Check sheet for the modelled part. Datum: model origin and axes. Units: mm. Face numbers are marked on the shaded views. A direction names the side the tool comes from. Round coordinates to 2 decimals unless told otherwise and drop trailing zeros. One line per item, written item: value. Start each with the question number.
1. Go/stop test with flat-tipped pins: pin 1 (3 mm diameter, centred on x = 4, z = 2.5, fed in from +Y); pin 2 (0.6 mm diameter, centred on x = 2.5, y = -7, fed in from -Z); pin 3 (1.5 mm diameter, centred on y = 2, z = 1.5, fed in from -X). Record where each tip stops, or that it passes through.
2. Material ranges on L1, parallel to Z at x = -5.25, y = -8; L2, parallel to X at y = 0.75, z = 4; L3, parallel to Y at x = 0, z = -0.9, recorded low to high.
3. Set-up check for the marked faces 1, 2 and 3: record each of +Z, -Z, +X, -X, +Y, -Y from which the full face is reachable in a straight line by a thin tool's end or side.
4. Release check for a two-part mould opening along X. For the marked faces 4, 5 and 6 record: +X half, -X half, draft (parallel to the pull), parting line (faces both ways), or undercut.
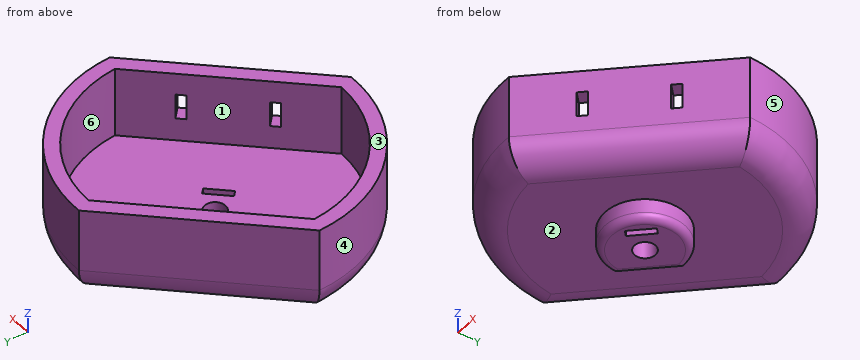
from build123d import *

# Parameters (mm, degrees)
BOSS_EXTRUDE1_DEPTH = 5
BOSS_EXTRUDE2_START = 1.5
BOSS_EXTRUDE2_DEPTH = 1.5
FILLET1_R           = 2
BOSS_EXTRUDE3_DEPTH = 1.5
SKETCH4_R           = 0.75
CUT_EXTRUDE1_DEPTH  = 17.248076932
SKETCH5_W           = 1.787924943
SKETCH5_H           = 0.660460042
CUT_EXTRUDE2_DEPTH  = 1
FILLET2_R           = 0.5


with BuildPart() as part:
    # Sketch1 → Boss-Extrude1 (new body)
    with BuildSketch(Plane.XY):
        with BuildLine():
            Line((0, 10), (-9.999822986, 0.0595))
            ThreePointArc((-9.999822986, 0.0595), (-7.09207304, -7.05), (0, -10))
            Line((0, -10), (10, 0))
            ThreePointArc((10, 0), (7.071067812, 7.071067812), (0, 10))
        make_face()
        with BuildLine():
            Line((0.403373919, 8.990955983), (-8.993196905, -0.349870591))
            ThreePointArc((-8.993196905, -0.349870591), (-6.383472043, -6.344390016), (-0.405092287, -8.990878725))
            Line((-0.405092287, -8.990878725), (8.990878725, 0.405092287))
            ThreePointArc((8.990878725, 0.405092287), (6.363352853, 6.36456915), (0.403373919, 8.990955983))
        make_face(mode=Mode.SUBTRACT)
    extrude(amount=BOSS_EXTRUDE1_DEPTH)

    # Sketch2 → Boss-Extrude2 (add)
    with BuildSketch(Plane(origin=(0, 0, 0), x_dir=(-1, 0, 0), z_dir=(0, 0, -1)).offset(BOSS_EXTRUDE2_START)):
        with BuildLine():
            Line((0, 10), (9.999822986, 0.0595))
            ThreePointArc((9.999822986, 0.0595), (7.09207304, -7.05), (0, -10))
            Line((0, -10), (-10, 0))
            ThreePointArc((-10, 0), (-7.071067812, 7.071067812), (0, 10))
        make_face()
    extrude(amount=-BOSS_EXTRUDE2_DEPTH)

    # Fillet1
    fillet1_edges = [part.edges().sort_by_distance(p)[0] for p in [
        (7.071067812, 7.071067812, -1.5),
        (5, -5, -1.5),
        (-7.09207304, -7.05, -1.5),
        (-4.999911493, 5.02975, -1.5),
    ]]
    fillet(fillet1_edges, radius=FILLET1_R)

    # Sketch3 → Boss-Extrude3 (add)
    with BuildSketch(Plane(origin=(0, 0, -1.5), x_dir=(-1, 0, 0), z_dir=(0, 0, -1))):
        with BuildLine():
            Line((0, 2.854684063), (2.854684063, 0))
            ThreePointArc((2.854684063, 0), (-2.018566459, -2.018566459), (0, 2.854684063))
        make_face()
    extrude(amount=BOSS_EXTRUDE3_DEPTH)

    # Sketch4 → Cut-Extrude1 (cut, through all)
    with BuildSketch(Plane(origin=(0, 0, -3), x_dir=(-1, 0, 0), z_dir=(0, 0, -1))):
        Circle(SKETCH4_R)
        Polygon((-1.673451771, -0.345114688), (-0.345114688, -1.673451771), (-0.677198959, -2.005536042), (-2.005536042, -0.677198959), align=None)
    extrude(amount=-CUT_EXTRUDE1_DEPTH, mode=Mode.SUBTRACT)

    # Sketch5 → Cut-Extrude2 (cut)
    with BuildSketch(Plane(origin=(5, -5, 0), x_dir=(0, 0, -1), z_dir=(0.7071067811865477, -0.7071067811865475, 0))):
        with Locations((-2.538538979, -2.770235161)):
            Rectangle(SKETCH5_W, SKETCH5_H)
        with Locations((-2.538538979, 2.770235161)):
            Rectangle(SKETCH5_W, SKETCH5_H)
    extrude(amount=-CUT_EXTRUDE2_DEPTH, mode=Mode.SUBTRACT)

    # Fillet2
    fillet2_edges = [part.edges().sort_by_distance(p)[0] for p in [
        (2.018566459, -2.018566459, -3),
        (-1.427342031, 1.427342031, -3),
    ]]
    fillet(fillet2_edges, radius=FILLET2_R)


solid = part.part
Taken from the geometry:
1. pin 1: stops at y = 9.68
1. pin 2: stops at z = -0.98
1. pin 3: stops at x = -8.8
2. L1: z = -0.74 to 5
2. L2: x = -9.31 to -7.89, 8.97 to 9.97
2. L3: y = -9.19 to -0.75, 0.75 to 9.19
3. face 1: +Z
3. face 2: -Z
3. face 3: +Z, +X, -X, +Y, -Y
4. face 4: -X half
4. face 5: +X half
4. face 6: undercut
